from build123d import *

# Parameters (mm, degrees)
F0_R     = 10.95
F1_DEPTH = 4
F2_SIZE  = 2


with BuildPart() as f1:
    # F0 (on Top) → F1 (new body, symmetric)
    with BuildSketch(Plane.XY):
        with BuildLine():
            Line((38.971143, -17.5), (4.330127, 42.5))
            ThreePointArc((4.330127, 42.5), (0, 45), (-4.330127, 42.5))
            Line((-4.330127, 42.5), (-38.971143, -17.5))
            ThreePointArc((-38.971143, -17.5), (-38.971143, -22.5), (-34.641016, -25))
            Line((-34.641016, -25), (34.641016, -25))
            ThreePointArc((34.641016, -25), (38.971143, -22.5), (38.971143, -17.5))
        make_face()
        Polygon((-18.258702, -21.675), (-27.900452, -21.675), (-32.721327, -13.325), (-27.900452, -4.975), (-18.258702, -4.975), (-13.437828, -13.325), align=None, mode=Mode.SUBTRACT)
        Circle(F0_R, mode=Mode.SUBTRACT)
        Polygon((27.900452, -4.975), (32.721327, -13.325), (27.900452, -21.675), (18.258702, -21.675), (13.437828, -13.325), (18.258702, -4.975), align=None, mode=Mode.SUBTRACT)
        Polygon((9.641749, 26.65), (4.820875, 18.3), (-4.820875, 18.3), (-9.641749, 26.65), (-4.820875, 35), (4.820875, 35), align=None, mode=Mode.SUBTRACT)
    extrude(amount=F1_DEPTH, both=True)

    # F2
    f2_edges = [f1.edges().sort_by_distance(p)[0] for p in [
        (-21.650635, 12.5, 4),
        (21.650635, 12.5, 4),
        (-21.650635, 12.5, -4),
    ]]
    chamfer(f2_edges, length=F2_SIZE)


solid = f1.part
Part model, mm, in its own coordinate system. A direction names the side the tool comes from. Coordinates: 2 decimals unless noted, no trailing zeros. Loops run counter-clockwise (first coordinate to the right, second up) from the corner with the lowest first, then second, coordinate; pieces in that order, holes last. Notation, with made-up numbers: (85, -10) -> (111, -10) arc R18 ccw to (111, 4) -> close; hole circle Ø7 at (72.5, 67.25). An arc over 180 degrees is marked (long way). Use a Markdown table: item, result. Add a question column.
Item 1: Band-saw the part on C-C on z = -0.25. Write the cut outline in (x, y) (3 decimals), plus the area to 3 significant figures.
Item 2: Band-saw the part on A-A on x = 0. Write the cut outline in (y, z).
Item 3: Band-saw the part on D-D on x = 14.5. Write the cut outline in (y, z).
Item 4: Probe probe 1 along Y at (x, z) = (6.5, -0.5); probe 2 along Y at (x, z) = (-8, -0.5); probe 3 along Y at (x, z) = (-19, -3.5) (3 decimals). List the from-to ranges inside material, lowest first.
Item 5: Band-saw the part on B-B on y = 0. Write the cut outline in (x, z), plus the area to 3 significant figures.
Item 6: Flat gauge pins, fed straight in: P1, Ø2, axis at y = 25.5, z = -0.5, coming from the -X side; P2, Ø19.5, axis at x = 0, y = 0, coming from the -Z side; P3, Ø4, axis at x = -22.5, z = 0, coming from the +Y side. Where does each tip first touch, or does it go through?
Item 7: Pull direction X, two halves, no side cores. Call faces 3 (the flat face through (-20.53, 12.413, 3.014)), 4 (the flat face through (21.893, 12.08, 0.028)), 5 (the flat face through (-15.882, -9.092, 0.056)): +X half, -X half, draft (parallel to the pull), parting line (faces both ways), or undercut.
Item 8: Which spindle directions (+Z, -Z, +X, -X, +Y, -Y) get a long thin tool onto all of the face, cutting with end or side? Do faces 1 (the cylindrical face through (38.934, -22.563, 0.028)), 2 (the flat face through (-30.277, -17.558, 0.056)). Say none if no direction does.
Geometry says:
| question | item | result |
|---|---|---|
| 1 | outline | (-38.971, -17.5) arc R5 ccw to (-34.641, -25) -> (34.641, -25) arc R5 ccw to (38.971, -17.5) -> (4.33, 42.5) arc R5 ccw to (-4.33, 42.5) -> close; hole (-32.721, -13.325) -> (-27.9, -21.675) -> (-18.259, -21.675) -> (-13.438, -13.325) -> (-18.259, -4.975) -> (-27.9, -4.975) -> close; hole circle Ø21.9 at (0, 0); hole (-9.642, 26.65) -> (-4.821, 18.3) -> (4.821, 18.3) -> (9.642, 26.65) -> (4.821, 35) -> (-4.821, 35) -> close; hole (13.438, -13.325) -> (18.259, -21.675) -> (27.9, -21.675) -> (32.721, -13.325) -> (27.9, -4.975) -> (18.259, -4.975) -> close |
| 1 | area | 2,090 mm² |
| 2 | outline | (-25, -2) -> (-23, -4) -> (-10.95, -4) -> (-10.95, 4) -> (-23, 4) -> (-25, 2) -> close; (10.95, -4) -> (18.3, -4) -> (18.3, 4) -> (10.95, 4) -> close; (35, -4) -> (43, -4) -> (45, -2) -> (45, 2) -> (43, 4) -> (35, 4) -> close |
| 3 | outline | (-25, -2) -> (-23, -4) -> (-15.16, -4) -> (-15.16, 4) -> (-23, 4) -> (-25, 2) -> close; (-11.49, -4) -> (20.89, -4) -> (24.89, -2) -> (24.89, 2) -> (20.89, 4) -> (-11.49, 4) -> close |
| 4 | probe 1 | -25 to -8.81, 8.81 to 21.21, 32.09 to 38.74 |
| 4 | probe 2 | -25 to -7.48, 7.48 to 23.81, 29.49 to 36.14 |
| 4 | probe 3 | -23.5 to -21.675, -4.975 to 14.091 |
| 5 | outline | (-28.87, -2) -> (-26.56, -4) -> (-10.95, -4) -> (-10.95, 4) -> (-26.56, 4) -> (-28.87, 2) -> close; (10.95, -4) -> (26.56, -4) -> (28.87, -2) -> (28.87, 2) -> (26.56, 4) -> (10.95, 4) -> close |
| 5 | area | 277 mm² |
| 6 | P1 | x = -14.72 |
| 6 | P2 | through |
| 6 | P3 | y = 14.49 |
| 7 | face 3 | -X half |
| 7 | face 4 | +X half |
| 7 | face 5 | undercut |
| 8 | face 1 | +Z, -Z, +X |
| 8 | face 2 | +Z, -Z |
